```python
from build123d import *

# Parameters (mm, degrees)
F1_DEPTH = 6
F2_W     = 14
F2_H     = 6
F2_W_2   = 4
F3_DEPTH = 8
F5_DEPTH = 3
F6_R     = 0.5


with BuildPart() as f1:
    # F0 (on Front) → F1 (new body, symmetric)
    with BuildSketch(Plane.XZ):
        with BuildLine():
            Line((-28, 0), (0, 0))
            Line((0, 0), (0, 10.75))
            Line((0, 10.75), (-4, 10.75))
            Line((-4, 10.75), (-4, 4))
            Line((-4, 4), (-18, 4))
            Line((-18, 4), (-18, 8))
            Line((-18, 8), (-21, 8))
            Line((-21, 8), (-21, 6))
            ThreePointArc((-21, 6), (-23, 4), (-25, 6))
            Line((-25, 6), (-25, 8))
            Line((-25, 8), (-28, 8))
            Line((-28, 8), (-28, 0))
        make_face()
    extrude(amount=F1_DEPTH, both=True)

    # F2 (on face) → F3 (cut)
    with BuildSketch(Plane.XY.offset(10.75)):
        with Locations((-11, 0)):
            Rectangle(F2_W, F2_H)
        with Locations((-2, 0)):
            Rectangle(F2_W_2, F2_H)
    extrude(amount=-F3_DEPTH, mode=Mode.SUBTRACT)

    # F4 (on Front) → F5 (join, symmetric)
    with BuildSketch(Plane.XZ):
        with BuildLine():
            Line((-12.3, 2.75), (0, 2.75))
            ThreePointArc((0, 2.75), (-3.916003, 4.928739), (-8.3, 4))
            ThreePointArc((-8.3, 4), (-10.466716, 3.90849), (-12.3, 2.75))
        make_face()
    extrude(amount=F5_DEPTH, both=True)

    # F6
    f6_edges = [f1.edges().sort_by_distance(p)[0] for p in [
        (-21, 0, 8),
        (-25, 0, 8),
        (-28, 0, 8),
        (-18, 0, 8),
        (0, -4.5, 10.75),
        (0, 4.5, 10.75),
        (-4, 4.5, 10.75),
        (-4, -4.5, 10.75),
    ]]
    fillet(f6_edges, radius=F6_R)


solid = f1.part
```
The listing builds one solid part. Answer for the finished solid, in the listing's coordinates (mm). A direction names the side the tool comes from. Give positions to 0.01 mm unless a question says otherwise; leave off trailing zeros. Loops run counter-clockwise (first coordinate to the right, second up) from the corner with the lowest first, then second, coordinate; pieces in that order, holes last. Notation, with made-up numbers: M 8,66.25 L 21,66.25 A16 ccw 21,81.25 Z; hole C 63,74.25 d8. An arc over 180 degrees is marked long. One line per item, written item: value.
Q1. A cutting plane is placed at A-A on y = 2.5. Determine the outline of the cut face in (x, z), then the cut area to 3 significant figures.
Working result:
outline: M -28,0 L 0,0 L 0,2.75 A6.39 ccw -8.3,4 A4.21 ccw -12.3,2.75 L -18,2.75 L -18,7.5 A0.5 ccw -18.5,8 L -20.5,8 A0.5 ccw -21,7.5 L -21,6 A2 cw -25,6 L -25,7.5 A0.5 ccw -25.5,8 L -27.5,8 A0.5 ccw -28,7.5 Z
area: 133 mm^2
Q2. A cutting plane is placed at C-C on y = 5. Determine the outline of the cut face in (x, z), then the cut area to 3 significant figures.
Working result:
outline: M -28,0 L 0,0 L 0,10.25 A0.5 ccw -0.5,10.75 L -3.5,10.75 A0.5 ccw -4,10.25 L -4,4 L -18,4 L -18,7.5 A0.5 ccw -18.5,8 L -20.5,8 A0.5 ccw -21,7.5 L -21,6 A2 cw -25,6 L -25,7.5 A0.5 ccw -25.5,8 L -27.5,8 A0.5 ccw -28,7.5 Z
area: 164 mm^2
Q3. Find the intervals of material crossed by line 1 (X direction, y = 5, z = 4.75); line 2 (X direction, y = 0.5, z = 4.5); line 3 (X direction, y = 1.5, z = 6.75), in increasing order. Write a range as from..to.
Working result:
line 1: x = -28..-24.56, -21.44..-18, -4..0
line 2: x = -28..-24.32, -21.68..-18, -7.35..-2.39
line 3: x = -28..-25, -21..-18
Q4. Flat-ended cylindrical pins translate along their axes: P1, Ø1.7, axis at x = -16.5, y = 1, coming from the +Z side; P2, Ø0.6, axis at x = -26, y = -1, coming from the +Z side; P3, Ø0.9, axis at x = -13.5, y = 5, coming from the +Z side. Find the tip coordinate at first contact, or state that the pin passes through.
Working result:
P1: stops at z = 2.75
P2: stops at z = 8
P3: stops at z = 4
Q5. For faces 4 (the face through (-26, 0, 8)), 5 (the face through (-2, 3, 8)), 6 (the face through (-11, 4, 4)), 7 (the face through (-21, 0, 7)), 8 (the face through (-10.437, -0.042, 3.918)), determine the directions among +Z, -Z, +X, -X, +Y, -Y from which every point of the face is accessible in a straight line to the end or side of a thin tool.
Working result:
face 4: +Z, -X, +Y, -Y
face 5: +Z, +X
face 6: +Z, +Y
face 7: +Z, +Y, -Y
face 8: +Z
Q6. A cutting plane is placed at D-D on x = -23. Determine the outline of the cut face in (y, z).
Working result:
outline: M -6,0 L 6,0 L 6,4 L -6,4 Z
Q7. Determine the mould class of faces 1 (the face through (-5.7, -3, 4.4)), 2 (the face through (-15, 3, 3)), 3 (the face through (-23, 0, 4)) for opening direction Y: +Y half, -Y half, draft (parallel to the pull), parting line (faces both ways), or undercut.
Working result:
face 1: -Y half
face 2: undercut
face 3: draft
Q8. A cutting plane is placed at B-B on x = -16.25. Determine the outline of the cut face in (y, z).
Working result:
outline: M -6,0 L 6,0 L 6,4 L 3,4 L 3,2.75 L -3,2.75 L -3,4 L -6,4 Z
